```python
from build123d import *

# Parameters (mm, degrees)
SKETCH1_R           = 50
SKETCH1_R_2         = 4
BOSS_EXTRUDE1_DEPTH = 12
SKETCH2_R           = 30
CUT_EXTRUDE1_DEPTH  = 72.721684308
CUT_EXTRUDE2_DEPTH  = 72.721684308
CHAMFER1_SIZE       = 7.819775181
CIRPATTERN1_DEPTH   = 12
FILLET1_R           = 4
BOSS_EXTRUDE2_START = 12
SKETCH4_R           = 4
BOSS_EXTRUDE2_DEPTH = 12
SKETCH5_R           = 8
CUT_EXTRUDE3_DEPTH  = 12


with BuildPart() as part:
    # Sketch1 → Boss-Extrude1 (new body)
    with BuildSketch(Plane.XY):
        Circle(SKETCH1_R)
        Circle(SKETCH1_R_2, mode=Mode.SUBTRACT)
    extrude(amount=BOSS_EXTRUDE1_DEPTH)

    # Sketch2 → Cut-Extrude1 (cut, through all)
    with BuildSketch(Plane.XY.offset(12)):
        with Locations((-70.710678119, 0)):
            Circle(SKETCH2_R)
    extrude(amount=-CUT_EXTRUDE1_DEPTH, mode=Mode.SUBTRACT)

    # Sketch3 → Cut-Extrude2 (cut, through all)
    with BuildSketch(Plane.XY.offset(12)):
        with BuildLine():
            Line((-32.526911935, 38.183766184), (-11.313708499, 16.970562748))
            ThreePointArc((-11.313708499, 16.970562748), (-11.313708499, 11.313708499), (-16.970562748, 11.313708499))
            Line((-16.970562748, 11.313708499), (-38.183766184, 32.526911935))
            ThreePointArc((-38.183766184, 32.526911935), (-38.183766184, 38.183766184), (-32.526911935, 38.183766184))
        make_face()
    extrude(amount=-CUT_EXTRUDE2_DEPTH, mode=Mode.SUBTRACT)

    # Chamfer1
    # the kernel refuses this chamfer: 7.819775181, 2 mm, written as the material it takes off along each edge
    with BuildSketch(Plane(origin=(-38.070447498, 32.413593249, 32.307159288), x_dir=(-0.6329652069887249, -0.7741802417665543, 0), z_dir=(0, 0, -1))) as chamfer1_piece_1:
        with BuildLine():
            Line((1.993389554, 0), (CHAMFER1_SIZE * 0.0998541086907, -CHAMFER1_SIZE * 0.995002088869))
            Line((CHAMFER1_SIZE * 0.0998541086907, -CHAMFER1_SIZE * 0.995002088869), (0, 0))
            ThreePointArc((0, 0), (1.020707521, 0.009929226), (1.993389554, 0))
        make_face()
    extrude(amount=52.614318575, mode=Mode.SUBTRACT)
    with BuildSketch(Plane(origin=(-32.413593249, 38.070447498, 32.307159288), x_dir=(0.7741802417665462, 0.6329652069887348, 0), z_dir=(0, 0, -1))) as chamfer1_piece_2:
        with BuildLine():
            Line((1.993389554, 0), (CHAMFER1_SIZE * 0.0998541086907, CHAMFER1_SIZE * 0.995002088869))
            Line((CHAMFER1_SIZE * 0.0998541086907, CHAMFER1_SIZE * 0.995002088869), (0, 0))
            ThreePointArc((0, 0), (1.020707521, -0.009929226), (1.993389554, 0))
        make_face()
    extrude(amount=52.614318575, mode=Mode.SUBTRACT)

    # CirPattern1: read off the stored shape, not the designer's step
    # CirPattern1 outline → CirPattern1 (cut)
    with BuildSketch(Plane.XY):
        with BuildLine():
            Line((39.33219373, -30.870350442), (32.541031441, -26.884177191))
            Line((32.541031441, -26.884177191), (16.970562748, -11.313708499))
            ThreePointArc((16.970562748, -11.313708499), (11.313708499, -11.313708499), (11.313708499, -16.970562748))
            Line((11.313708499, -16.970562748), (26.884177191, -32.541031441))
            Line((26.884177191, -32.541031441), (30.870350442, -39.33219373))
            ThreePointArc((30.870350442, -39.33219373), (35.355339059, -35.355339059), (39.33219373, -30.870350442))
        make_face()
        with BuildLine():
            ThreePointArc((-17.944358445, 46.669047558), (0, 40.710678119), (17.944358445, 46.669047558))
            ThreePointArc((17.944358445, 46.669047558), (0, 50), (-17.944358445, 46.669047558))
        make_face()
        with BuildLine():
            Line((32.541031441, 26.884177191), (39.33219373, 30.870350442))
            ThreePointArc((39.33219373, 30.870350442), (35.35533906, 35.35533906), (30.870350442, 39.33219373))
            Line((30.870350442, 39.33219373), (26.884177191, 32.541031441))
            Line((26.884177191, 32.541031441), (11.313708499, 16.970562748))
            ThreePointArc((11.313708499, 16.970562748), (11.313708499, 11.313708499), (16.970562748, 11.313708499))
            Line((16.970562748, 11.313708499), (32.541031441, 26.884177191))
        make_face()
        with BuildLine():
            ThreePointArc((46.669047558, 17.944358445), (40.710678119, 0), (46.669047558, -17.944358445))
            ThreePointArc((46.669047558, -17.944358445), (50, 0), (46.669047558, 17.944358445))
        make_face()
        with BuildLine():
            ThreePointArc((-39.33219373, -30.870350442), (-35.355339059, -35.355339059), (-30.870350442, -39.332193729))
            Line((-30.870350442, -39.332193729), (-26.884177191, -32.541031441))
            Line((-26.884177191, -32.541031441), (-11.313708499, -16.970562748))
            ThreePointArc((-11.313708499, -16.970562748), (-11.313708499, -11.313708499), (-16.970562748, -11.313708499))
            Line((-16.970562748, -11.313708499), (-32.541031441, -26.884177191))
            Line((-32.541031441, -26.884177191), (-39.33219373, -30.870350442))
        make_face()
        with BuildLine():
            ThreePointArc((-17.944358445, -46.669047558), (0, -50), (17.944358445, -46.669047558))
            ThreePointArc((17.944358445, -46.669047558), (0, -40.710678119), (-17.944358445, -46.669047558))
        make_face()
    extrude(amount=CIRPATTERN1_DEPTH, mode=Mode.SUBTRACT)

    # Fillet1
    fillet1_edges = [part.edges().sort_by_distance(p)[0] for p in [
        (-46.669047558, -17.944358445, 6),
        (-46.669047558, 17.944358445, 6),
        (17.944358445, 46.669047558, 6),
        (-17.944358445, 46.669047558, 6),
        (46.669047558, -17.944358445, 6),
        (46.669047558, 17.944358445, 6),
        (-17.944358445, -46.669047558, 6),
        (17.944358445, -46.669047558, 6),
    ]]
    fillet(fillet1_edges, radius=FILLET1_R)

    # Sketch4 → Boss-Extrude2 (add)
    with BuildSketch(Plane(origin=(0, 0, 0), x_dir=(-1, 0, 0), z_dir=(0, 0, -1)).offset(BOSS_EXTRUDE2_START)):
        with BuildLine():
            Line((12.990381057, -7.5), (8.660254038, -15))
            ThreePointArc((8.660254038, -15), (0, -20), (-8.660254038, -15))
            Line((-8.660254038, -15), (-12.990381057, -7.5))
            ThreePointArc((-12.990381057, -7.5), (0, 15), (12.990381057, -7.5))
        make_face()
        Circle(SKETCH4_R, mode=Mode.SUBTRACT)
    extrude(amount=-BOSS_EXTRUDE2_DEPTH)

    # Sketch5 → Cut-Extrude3 (cut)
    with BuildSketch(Plane.XY.offset(12)):
        Circle(SKETCH5_R)
    extrude(amount=-CUT_EXTRUDE3_DEPTH, mode=Mode.SUBTRACT)


solid = part.part
```
Geometry check sheet. Reference: the model listing, model coordinates, mm. A direction names the side the tool comes from. Round coordinates to 2 decimals unless told otherwise and drop trailing zeros. Loops run counter-clockwise (first coordinate to the right, second up) from the corner with the lowest first, then second, coordinate; pieces in that order, holes last. Notation, with made-up numbers: M 76.25,49 L 104.25,49 A35 ccw 104.25,87 Z; hole C 16,54 d6. An arc over 180 degrees is marked long. Return JSON: item names as keys, results as strings. Group by question number.
(1) Mould release check, pull along X, two halves, no side actions. Record for faces 1 (the face through (-10.856, -11.198, -6.084)), 2 (the face through (40.71, 0.24, 5.92)), 3 (the face through (-35.89, -28.85, 5.92)), 4 (the face through (-11.25, 11.38, 6.08)): pulls with the +X half, pulls with the -X half, needs draft (parallel to the pull), parting line crosses it, or undercut.
(2) Set-up check for faces 5 (the face through (24.865, -19.208, 5.916)), 6 (the face through (10.795, -11.302, -6.084)), 7 (the face through (-35.984, 28.905, 6.084)): record each of +Z, -Z, +X, -X, +Y, -Y from which the full face is reachable in a straight line by a thin tool's end or side.
(3) Section check D-D, the plane y = -23. Enter the section's corners in (x, z), and give its area (3 significant figures).
(4) Section check B-B, the plane y = 0. Enter the section's corners in (x, z).
(5) Go/stop test with flat-tipped pins: pin 1 (1.5 mm diameter, centred on x = -16.5, z = 0, fed in from -Y); pin 2 (13 mm diameter, centred on x = 0, y = 0, fed in from +Z); pin 3 (5 mm diameter, centred on x = 0, y = 0, fed in from -Z) (3 decimals); pin 4 (10 mm diameter, centred on x = 5, z = -7, fed in from +Y). Record where each tip stops, or that it passes through.
(6) Scan lines: line 1 along X through (y, z) = (0, -10.5); line 2 along X through (y, z) = (-14, 4.75); line 3 along Z through (x, y) = (-7, -26). Record each from-to range of solid material in increasing order. Write a range as [from, to].
(7) Section check A-A, the plane x = 0. Enter the section's corners in (y, z), and give its area (3 significant figures).
(8) Section check C-C, the plane z = -5.25. Enter the section's corners in (x, y).
Data:
{
 "1": {"face 1": "pulls with the -X half", "face 2": "pulls with the +X half", "face 3": "undercut", "face 4": "undercut"},
 "2": {"face 5": "+Z, -Z", "face 6": "-Z, +X, -Y", "face 7": "+Z, -Z, +Y"},
 "3": {"outline": "M -44.4,0 L -28.66,0 L -28.66,12 L -44.4,12 Z; M -17.34,0 L 17.34,0 L 17.34,12 L -17.34,12 Z; M 28.66,0 L 44.4,0 L 44.4,12 L 28.66,12 Z", "area": "794 mm²"},
 "4": {"outline": "M -40.71,0 L -15,0 L -15,-12 L -4,-12 L -4,0 L -8,0 L -8,12 L -40.71,12 Z; M 4,-12 L 15,-12 L 15,0 L 40.71,0 L 40.71,12 L 8,12 L 8,0 L 4,0 Z"},
 "5": {"pin 1": "y = -45.96", "pin 2": "z = 0", "pin 3": "through", "pin 4": "y = 15"},
 "6": {"line 1": "[-15, -4], [4, 15]", "line 2": "[-44.18, -19.66], [-10.14, 10.14], [19.66, 44.18]", "line 3": "[0, 12]"},
 "7": {"outline": "M -40.71,0 L -20,0 L -20,-12 L -4,-12 L -4,0 L -8,0 L -8,12 L -40.71,12 Z; M 4,-12 L 15,-12 L 15,0 L 40.71,0 L 40.71,12 L 8,12 L 8,0 L 4,0 Z", "area": "1,110 mm²"},
 "8": {"outline": "M -12.99,-7.5 L -8.66,-15 A10 ccw 8.66,-15 L 12.99,-7.5 A15 ccw long Z; hole C 0,0 d8"}
}
